```python
from build123d import *

# Parameters (mm, degrees)
ESBO_O1_R                  = 12.5
ESBO_O1_R_2                = 10
RESSALTO_EXTRUS_O1_DEPTH   = 180
CORTE_EXTRUS_O1_DEPTH      = 5
CORTE_EXTRUS_O1_DEPTH_BACK = 5
ESBO_O2_R                  = 12.5
ESBO_O2_R_2                = 12


with BuildPart() as part:
    # Esbo_o1 → Ressalto-extrus_o1 (new body)
    with BuildSketch(Plane.XY):
        with Locations(Location((0, 0, 0), (0, 0, 180))):
            Circle(ESBO_O1_R)
        with Locations(Location((0, 0, 0), (0, 0, 180))):
            Circle(ESBO_O1_R_2, mode=Mode.SUBTRACT)
    extrude(amount=RESSALTO_EXTRUS_O1_DEPTH)

    # Esbo_o2 → Corte-extrus_o1 (cut, two sides: drawn at the far end of the back side and taken through both)
    with BuildSketch(Plane(origin=(0, 0, 0), x_dir=(0, 0, -1), z_dir=(1, 0, 0)).offset(-CORTE_EXTRUS_O1_DEPTH_BACK)):
        with Locations((5, 0)):
            Circle(ESBO_O2_R)
        with Locations((5, 0)):
            Circle(ESBO_O2_R_2, mode=Mode.SUBTRACT)
    extrude(amount=CORTE_EXTRUS_O1_DEPTH + CORTE_EXTRUS_O1_DEPTH_BACK, mode=Mode.SUBTRACT)


solid = part.part
```
The model under review builds one solid part; all positions refer to its coordinate system, in mm. A direction names the side the tool comes from. Round coordinates to 2 decimals unless told otherwise and drop trailing zeros. Write each loop counter-clockwise with the first axis right and the second up, starting at its lowest first coordinate (ties: lowest second). Pieces come first, ordered by that corner, then holes. Notation, with made-up numbers: (56, 80) - (91, 80) arc R17 ccw to (91, 91) - close; hole circle Ø9 at (-27, 79.25). An arc over 180 degrees is marked (long way). One line per question, with ' | ' between items.
Item 1: For faces 1 (the face through (-5, 10, 2)), 2 (the face through (10, 0, 89)), list the 3-axis set-ups (+Z, -Z, +X, -X, +Y, -Y) from which the entire face can be reached by the end or side of a thin tool; tool diameter is ignored.
Resolved:
face 1: none | face 2: +Z, -Z
Item 2: For P1, Ø5, axis at y = 9, z = 140.5, coming from the +X side; P2, Ø3, axis at x = 3.5, z = 21.5, coming from the +Y side; P3, Ø1, axis at y = -7.5, z = 76.5, coming from the -X side, all flat-tipped, find the tip position at first contact; note any pin that passes through.
Resolved:
P1: stops at x = 10.68 | P2: stops at y = 12.34 | P3: stops at x = -10.36
Item 3: Add section B-B, the plane x = 7.25. Give the boundary of the cut face in (y, z).
Resolved:
outline: (-10.18, 0) - (-6.89, 0) - (-6.89, 180) - (-10.18, 180) - close; (6.89, 0) - (10.18, 0) - (10.18, 180) - (6.89, 180) - close
Item 4: Add section A-A, the plane y = 0. Give the boundary of the cut face in (x, z), then the cut area to 3 significant figures.
Resolved:
outline: (-12.5, 0) - (-10, 0) - (-10, 180) - (-12.5, 180) - close; (10, 0) - (12.5, 0) - (12.5, 180) - (10, 180) - close | area: 900 mm2
Item 5: Add section C-C, the plane x = 0. Give the boundary of the cut face in (y, z).
Resolved:
outline: (-12.5, 0) - (-11.46, 0) arc R12.5 cw to (-10, 2.5) - (-10, 180) - (-12.5, 180) - close; (-10.91, 0) - (-10, 0) - (-10, 1.63) arc R12 ccw to start; (10, 0) - (10.91, 0) arc R12 ccw to (10, 1.63) - close; (10, 2.5) arc R12.5 cw to (11.46, 0) - (12.5, 0) - (12.5, 180) - (10, 180) - close
Item 6: To check wall thickness, follow probe 1 along Y at (x, z) = (0, 70); probe 2 along X at (y, z) = (7.5, 37); probe 3 along Y at (x, z) = (-3.5, 28.5). State the ranges of each line that lie inside material, in increasing order.
Resolved:
probe 1: y = -12.5 to -10, 10 to 12.5 | probe 2: x = -10 to -6.61, 6.61 to 10 | probe 3: y = -12 to -9.37, 9.37 to 12
Item 7: The part is to be moulded in two halves that separate along Z. For faces 3 (the face through (5, 10, 2)), 4 (the face through (-11.923, -3.755, 88.74)), 5 (the face through (7, -8, 0)), say which applies: pulls with the +Z half, pulls with the -Z half, needs draft (parallel to the pull), parting line crosses it, or undercut.
Resolved:
face 3: undercut | face 4: needs draft | face 5: pulls with the -Z half
Item 8: Add section D-D, the plane z = 160. Give the boundary of the cut face in (x, y).
Resolved:
outline: circle Ø25 at (0, 0); hole circle Ø20 at (0, 0)
